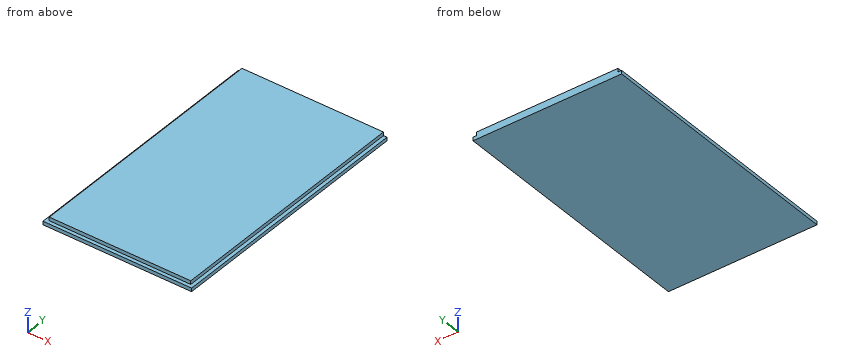
Autodesk Inventor part; units mm, degrees
ref_plane "YZ Plane" through (0, 0, 0) normal (1, 0, 0) x (0, 1, 0)
ref_plane "XZ Plane" through (0, 0, 0) normal (0, 1, 0) x (-1, 0, 0)
ref_plane "XY Plane" through (0, 0, 0) normal (0, 0, 1) x (1, 0, 0)
sketch "Sketch1" plane through (0, 0, 0) normal (0, 0, 1) x (1, 0, 0)
  line L0 (0, 217) -> (126, 217)
  line L1 (126, 217) -> (126, 0)
  line L2 (126, 0) -> (0, 0)
  line L3 (0, 0) -> (0, 217)
  dimension "d0" = 126
  dimension "d1" = 217
extrude "Extrusion1" add sketch "Sketch1" along normal blind 3
sketch "Sketch2" plane through (0, 0, 3) normal (0, 0, 1) x (1, 0, 0)
  line L0 (0, 0) -> (126, 0)
  line L1 (126, 0) -> (126, 217)
  line L2 (126, 217) -> (0, 217)
  line L3 (0, 217) -> (0, 0)
  line L4 (3, 217) -> (123, 217)
  line L5 (123, 217) -> (123, 3)
  line L6 (123, 3) -> (3, 3)
  line L7 (3, 3) -> (3, 217)
  dimension "d4" = 3
  dimension "d5" = 3
  dimension "d6" = 3
extrude "Extrusion2" add sketch "Sketch2" along normal blind 3 contours L2 L5 L6 L7
properties part number "Tapa pared falsa"
Source: CAD feature listing. Evaluate the final solid. Frame: model axes, mm. Coordinates: 2 decimals unless noted, no trailing zeros. Loops run counter-clockwise (first coordinate to the right, second up) from the corner with the lowest first, then second, coordinate; pieces in that order, holes last. Notation, with made-up numbers: (66, -12.75) -> (75, -12.75) arc R25 ccw to (75, 1.25) -> close; hole circle Ø1 at (-10.75, -21). An arc over 180 degrees is marked (long way). One line per item, written item: value. Start each with the question number.
Q1. Line query: line 1 along X through (y, z) = (135.5, 3.7); line 2 along Y through (x, z) = (96.5, 4.9). Output: solid intervals per line, ascending.
Q2. Section query B-B, the plane z = 4.4. Return the cut outline in (x, y).
Q3. Contact query for flat-ended pins moving along their axis: P1, Ø2, axis at x = 60, y = 141.5, coming from the -Z side; P2, Ø0.9, axis at x = 58, z = 5, coming from the -Y side; P3, Ø2.5, axis at y = 147.5, z = 5, coming from the +X side; P4, Ø2.5, axis at y = 79, z = 4.5, coming from the -X side. Output: stop coordinate, or through.
Q4. Section query A-A, the plane y = 161.5. Return the cut outline in (x, z), and give its area (3 significant figures).
Results:
1. line 1: 3 to 123
1. line 2: 3 to 217
2. outline: (3, 3) -> (123, 3) -> (123, 217) -> (3, 217) -> close
3. P1: z = 0
3. P2: y = 3
3. P3: x = 123
3. P4: x = 3
4. outline: (0, 0) -> (126, 0) -> (126, 3) -> (123, 3) -> (123, 6) -> (3, 6) -> (3, 3) -> (0, 3) -> close
4. area: 738 mm^2
